from build123d import *

# Parameters (mm, degrees)
CROQUIS1_W             = 50
CROQUIS1_H             = 85
BRIDA_BASE1_DEPTH      = 2
BRIDA_DE_ARISTA1_DEPTH = 85
DESDOBLAR1_START       = -42.5
DESDOBLAR1_DEPTH       = 85
DESDOBLAR1_2_DEPTH     = 85
CROQUIS9_W             = 49.2634
CROQUIS9_H             = 35
CROQUIS9_W_2           = 2.727844901
CORTAR_EXTRUIR1_DEPTH  = 10
DOBLAR1_START          = -7.5
DOBLAR1_DEPTH          = 50
DOBLAR1_2_DEPTH        = 50
DOBLAR1_START_2        = 27.727844901
DOBLAR1_3_DEPTH        = 50.272155099
DOBLAR1_START_3        = 25.7366
DOBLAR1_4_DEPTH        = 2
CROQUIS11_R            = 6
CROQUIS11_R_2          = 2.5
CORTAR_EXTRUIR2_DEPTH  = 10


with BuildPart() as part:
    # Brida base1: sheet metal written as solids
    # Croquis1 → Brida base1 (new body)
    with BuildSketch(Plane.XY):
        Rectangle(CROQUIS1_W, CROQUIS1_H)
    extrude(amount=-BRIDA_BASE1_DEPTH)

    # Brida de arista1: sheet metal written as solids
    # Brida de arista1 section (on a plane across the edge) → Brida de arista1 (add)
    with BuildSketch(Plane(origin=(25.7366, -42.5, 0), x_dir=(-1, 0, 0), z_dir=(0, 1, 0))):
        with BuildLine():
            Line((-2, 0.7366), (-2, 50))
            Line((-2, 50), (0, 50))
            Line((0, 50), (0, 0.7366))
            ThreePointArc((0, 0.7366), (0.215745145, 0.215745145), (0.7366, 0))
            Line((0.7366, 0), (0.7366, -2))
            ThreePointArc((0.7366, -2), (-1.198468417, -1.198468417), (-2, 0.7366))
        make_face()
    extrude(amount=BRIDA_DE_ARISTA1_DEPTH)

    # Desdoblar1: read off the stored shape, not the designer's step
    # Desdoblar1 outline → Desdoblar1 (cut)
    with BuildSketch(Plane(origin=(0, 0, 0), x_dir=(1, 0, 0), z_dir=(0, 1, 0)).offset(DESDOBLAR1_START)):
        with BuildLine():
            ThreePointArc((27.7366, -0.7366), (27.711233029, -0.364854094), (27.635602398, 0))
            Line((27.635602398, 0), (25, 0))
            ThreePointArc((25, 0), (25.520854855, -0.215745145), (25.7366, -0.7366))
            Line((25.7366, -0.7366), (25.7366, -50))
            Line((25.7366, -50), (27.7366, -50))
            Line((27.7366, -50), (27.7366, -0.7366))
        make_face()
    extrude(amount=DESDOBLAR1_DEPTH, mode=Mode.SUBTRACT)

    # Desdoblar1 2 outline → Desdoblar1 2 (add)
    with BuildSketch(Plane(origin=(0, 0, 0), x_dir=(1, 0, 0), z_dir=(0, 1, 0)).offset(DESDOBLAR1_START)):
        with BuildLine():
            Line((76.991244901, 2), (25, 2))
            ThreePointArc((25, 2), (26.654267209, 1.443395312), (27.635602398, 0))
            Line((27.635602398, 0), (76.991244901, 0))
            Line((76.991244901, 0), (76.991244901, 2))
        make_face()
    extrude(amount=DESDOBLAR1_2_DEPTH)

    # Croquis9 → Cortar-Extruir1 (cut)
    with BuildSketch(Plane.XY):
        Polygon((27.727844901, 39.876630521), (76.991244901, -7.5), (76.991244901, 42.5), (27.727844901, 42.5), align=None)
        with Locations((52.359544901, -25)):
            Rectangle(CROQUIS9_W, CROQUIS9_H)
        with Locations((26.36392245, -25)):
            Rectangle(CROQUIS9_W_2, CROQUIS9_H)
    extrude(amount=-CORTAR_EXTRUIR1_DEPTH, mode=Mode.SUBTRACT)

    # Doblar1: read off the stored shape, not the designer's step
    # Doblar1 outline → Doblar1 (cut)
    with BuildSketch(Plane(origin=(0, 0, 0), x_dir=(1, 0, 0), z_dir=(0, 1, 0)).offset(DOBLAR1_START)):
        with BuildLine():
            ThreePointArc((25, 2), (26.654267209, 1.443395312), (27.635602398, 0))
            Line((27.635602398, 0), (27.727844901, 0))
            Line((27.727844901, 0), (27.727844901, 2))
            Line((27.727844901, 2), (25, 2))
        make_face()
    extrude(amount=DOBLAR1_DEPTH, mode=Mode.SUBTRACT)

    # Doblar1 2 outline → Doblar1 2 (add)
    with BuildSketch(Plane(origin=(0, 0, 0), x_dir=(1, 0, 0), z_dir=(0, 1, 0)).offset(DOBLAR1_START)):
        with BuildLine():
            ThreePointArc((25, 0), (25.520854855, -0.215745145), (25.7366, -0.7366))
            Line((25.7366, -0.7366), (27.7366, -0.7366))
            ThreePointArc((27.7366, -0.7366), (27.711233029, -0.364854094), (27.635602398, 0))
            Line((27.635602398, 0), (25, 0))
        make_face()
    extrude(amount=DOBLAR1_2_DEPTH)

    # Doblar1 3 outline → Doblar1 3 (cut)
    with BuildSketch(Plane.YZ.offset(DOBLAR1_START_2)):
        Polygon((42.508419782, -2), (40.585019021, 0), (-7.5, 0), (-7.5, -2), align=None)
    extrude(amount=DOBLAR1_3_DEPTH, mode=Mode.SUBTRACT)

    # Doblar1 4 outline → Doblar1 4 (add)
    with BuildSketch(Plane.YZ.offset(DOBLAR1_START_3)):
        Polygon((-7.5, 50), (-7.5, 0.7366), (39.876630521, 0.7366), align=None)
    extrude(amount=DOBLAR1_4_DEPTH)

    # Croquis11 → Cortar-Extruir2 (cut)
    with BuildSketch(Plane.XY):
        with Locations((-13, 17.5)):
            Circle(CROQUIS11_R)
        with Locations((-13, -0.2)):
            Circle(CROQUIS11_R_2)
        with Locations((-13, 35.2)):
            Circle(CROQUIS11_R_2)
    extrude(amount=-CORTAR_EXTRUIR2_DEPTH, mode=Mode.SUBTRACT)


solid = part.part
Here's how the part is built. I have some questions about the finished solid (model axes, mm). A direction names the side the tool comes from. Give positions to 0.01 mm unless a question says otherwise; leave off trailing zeros. Order: outer loops, then holes, each group sorted by start corner. A loop starts at its lowest first (then second) coordinate and runs counter-clockwise, first axis right, second up. Notation, with made-up numbers: (76, -2) -> (117, -2) arc R13 cw to (117, 3) -> close; hole circle Ø5 at (88.25, 84.25). An arc over 180 degrees is marked (long way). Use a Markdown table: item, result. Add a question column.
Item 1: If we mould it in two halves opening along X, with no side actions, what happens to faces 1 (the face through (0, -1, 0)), 2 (the face through (-25, -1, -1)), 3 (the face through (-7.277, 19.302, -0.986))? For each: pulls with the +X half, pulls with the -X half, needs draft (parallel to the pull), parting line crosses it, or undercut.
Item 2: Imagine slicing it at A-A on x = -13. Please give me the cut outline in (y, z), plus the area to 3 significant figures.
Item 3: I need wall thicknesses on line 1 (Y direction, x = -13, z = -0.95); line 2 (Z direction, x = 10, y = -38); line 3 (X direction, y = 19.5, z = 3). Which ranges of each line are inside material? Lowest first, please.
Item 4: Imagine slicing it at B-B on y = -0.2. Please give me the cut outline in (x, z), plus the area to 3 significant figures.
Item 5: Imagine slicing it at D-D on x = -22. Please give me the cut outline in (y, z), plus the area to 3 significant figures.
Item 6: Will these pins go through, and if not, where does the flat tip stop? pin 1 (6.5 mm diameter, centred on x = -13, y = 35.2, fed in from +Z); pin 2 (2 mm diameter, centred on x = 26, z = 18, fed in from -Y); pin 3 (0.6 mm diameter, centred on x = 26.5, y = 41.5, fed in from +Z).
Item 7: For faces 4 (the face through (25.737, 5, 15)), 5 (the face through (27, 41, 0.737)), 6 (the face through (27.737, 5, 15)), 7 (the face through (-14.84, 36.89, -0.99)), 8 (the face through (25, -25, -1)), which set-ups out of +Z, -Z, +X, -X, +Y, -Y let a thin tool reach every point of the face, with its end or its side?
Item 8: Imagine slicing it at C-C on y = 9.5. Please give me the cut outline in (x, z).
Data:
| question | item | result |
|---|---|---|
| 1 | face 1 | needs draft |
| 1 | face 2 | pulls with the -X half |
| 1 | face 3 | undercut |
| 2 | outline | (-42.5, -2) -> (-2.7, -2) -> (-2.7, 0) -> (-42.5, 0) -> close; (2.3, -2) -> (11.5, -2) -> (11.5, 0) -> (2.3, 0) -> close; (23.5, -2) -> (32.7, -2) -> (32.7, 0) -> (23.5, 0) -> close; (37.7, -2) -> (42.5, -2) -> (42.5, 0) -> (37.7, 0) -> close |
| 2 | area | 126 mm² |
| 3 | line 1 | y = -42.5 to -2.7, 2.3 to 11.5, 23.5 to 32.7, 37.7 to 42.5 |
| 3 | line 2 | z = -2 to 0 |
| 3 | line 3 | x = 25.74 to 27.74 |
| 4 | outline | (-25, -2) -> (-15.5, -2) -> (-15.5, 0) -> (-25, 0) -> close; (-10.5, -2) -> (25, -2) arc R2.74 ccw to (27.74, 0.74) -> (27.74, 42.41) -> (25.74, 42.41) -> (25.74, 0.74) arc R0.74 cw to (25, 0) -> (-10.5, 0) -> close |
| 4 | area | 179 mm² |
| 5 | outline | (-42.5, -2) -> (42.5, -2) -> (42.5, 0) -> (-42.5, 0) -> close |
| 5 | area | 170 mm² |
| 6 | pin 1 | stops at z = 0 |
| 6 | pin 2 | stops at y = -7.5 |
| 6 | pin 3 | stops at z = 0.74 |
| 7 | face 4 | +Z, -X, +Y, -Y |
| 7 | face 5 | +Z, +X, -X, +Y |
| 7 | face 6 | +Z, -Z, +X, +Y, -Y |
| 7 | face 7 | +Z, -Z |
| 7 | face 8 | +Z, -Z, +X, -Y |
| 8 | outline | (-25, -2) -> (25, -2) arc R2.74 ccw to (27.74, 0.74) -> (27.74, 32.32) -> (25.74, 32.32) -> (25.74, 0.74) arc R0.74 cw to (25, 0) -> (-25, 0) -> close |
